Read the model definition and answer for the solid it produces. Units are mm, in the model's axes. A direction names the side the tool comes from. Coordinates: 2 decimals unless noted, no trailing zeros. Write each loop counter-clockwise with the first axis right and the second up, starting at its lowest first coordinate (ties: lowest second). Pieces come first, ordered by that corner, then holes. Notation, with made-up numbers: (-1.75, 30.5) -> (2.25, 30.5) arc R18 ccw to (2.25, 53.5) -> close; hole circle Ø4 at (-22, 39.5). An arc over 180 degrees is marked (long way). Answer as a JSON object with one key per item and string values. Group by question number.
(1) Find section D-D (x = 6.25). Give the vertices of the cut face in (y, z), then the cut area to 3 significant figures.
(2) Find section C-C (y = 3). Give the vertices of the cut face in (x, z), then the cut area to 3 significant figures.
(3) Find section B-B (x = -10). Give the vertices of the cut face in (y, z), then the cut area to 3 significant figures.
(4) Find section A-A (z = 18). Give the vertices of the cut face in (x, y).
(5) Flat-ended cylindrical pins translate along their axes: P1, Ø2, axis at x = 2.5, z = 11.5, coming from the +Y side; P2, Ø5, axis at x = 10, y = 3, coming from the +Z side. Find the tip coordinate at first contact, or state that the pin passes through.
(6) Straight lines are drawn through the part: L1, parallel to X at y = -12.65, z = 18; L2, parallel to Y at x = 10, z = 1.45; L3, parallel to Y at x = -5, z = 19.75. For each, find the intervals that lie inside material, in ascending order.
(7) Which of the six approach directions +Z, -Z, +X, -X, +Y, -Y give full straight-line access (tool end or side, diameter ignored) to faces 1 (the face through (0, 2, 3)), 2 (the face through (0, -13, 30))?
(8) For a pull along Z with two mould halves and no side action, classify faces 3 (the face through (0.21, -14.715, 0.301)), 4 (the face through (10.07, -13.48, 16.5)), 5 (the face through (0, -12, 17)), 6 (the face through (-9.93, -13.48, 16.5)) as +Z half, -Z half, draft (parallel to the pull), parting line (faces both ways), or undercut.
from build123d import *

# Parameters (mm, degrees)
SKETCH_1_W          = 30
SKETCH_1_H          = 30
EXTRUDE_1_DEPTH     = 3
SKETCH_2_R          = 1.5
CUT_EXTRUDE_1_DEPTH = 3.5
SKETCH_3_W          = 30
SKETCH_3_H          = 3
EXTRUDE_2_DEPTH     = 27
SKETCH_4_R          = 1.5
CUT_EXTRUDE_2_DEPTH = 27
FILLET_1_R          = 1
FILLET_2_R          = 1


with BuildPart() as part:
    # 草图1 → 凸台-拉伸1 (new body)
    with BuildSketch(Plane.XY):
        Rectangle(SKETCH_1_W, SKETCH_1_H)
    extrude(amount=EXTRUDE_1_DEPTH)

    # 草图2 → 切除-拉伸1 (cut)
    with BuildSketch(Plane.XY.offset(3)):
        with Locations((10, 3)):
            Circle(SKETCH_2_R)
        with Locations((-10, 3)):
            Circle(SKETCH_2_R)
    extrude(amount=-CUT_EXTRUDE_1_DEPTH, mode=Mode.SUBTRACT)

    # 草图3 → 凸台-拉伸2 (add)
    with BuildSketch(Plane.XY.offset(3)):
        with Locations((0, -13.5)):
            Rectangle(SKETCH_3_W, SKETCH_3_H)
    extrude(amount=EXTRUDE_2_DEPTH)

    # 草图4 → 切除-拉伸2 (cut)
    with BuildSketch(Plane(origin=(0, -12, 0), x_dir=(1, 0, 0), z_dir=(0, 1, 0))):
        with Locations(Location((10, -18, 0), (0, 0, 270))):
            Circle(SKETCH_4_R)
        with Locations(Location((-10, -18, 0), (0, 0, 270))):
            Circle(SKETCH_4_R)
    extrude(amount=-CUT_EXTRUDE_2_DEPTH, mode=Mode.SUBTRACT)

    # 圆角1
    fillet_1_edges = [part.edges().sort_by_distance(p)[0] for p in [
        (0, -12, 3),
    ]]
    fillet(fillet_1_edges, radius=FILLET_1_R)

    # 圆角2
    fillet_2_edges = [part.edges().sort_by_distance(p)[0] for p in [
        (0, -15, 0),
    ]]
    fillet(fillet_2_edges, radius=FILLET_2_R)


solid = part.part
Results below:
{
 "1": {"outline": "(-15, 1) arc R1 ccw to (-14, 0) -> (15, 0) -> (15, 3) -> (-11, 3) arc R1 cw to (-12, 4) -> (-12, 30) -> (-15, 30) -> close", "area": "171 mm2"},
 "2": {"outline": "(-15, 0) -> (-11.5, 0) -> (-11.5, 3) -> (-15, 3) -> close; (-8.5, 0) -> (8.5, 0) -> (8.5, 3) -> (-8.5, 3) -> close; (11.5, 0) -> (15, 0) -> (15, 3) -> (11.5, 3) -> close", "area": "72.0 mm2"},
 "3": {"outline": "(-15, 1) arc R1 ccw to (-14, 0) -> (1.5, 0) -> (1.5, 3) -> (-11, 3) arc R1 cw to (-12, 4) -> (-12, 16.5) -> (-15, 16.5) -> close; (-15, 19.5) -> (-12, 19.5) -> (-12, 30) -> (-15, 30) -> close; (4.5, 0) -> (15, 0) -> (15, 3) -> (4.5, 3) -> close", "area": "153 mm2"},
 "4": {"outline": "(-15, -15) -> (-11.5, -15) -> (-11.5, -12) -> (-15, -12) -> close; (-8.5, -15) -> (8.5, -15) -> (8.5, -12) -> (-8.5, -12) -> close; (11.5, -15) -> (15, -15) -> (15, -12) -> (11.5, -12) -> close"},
 "5": {"P1": "stops at y = -12", "P2": "stops at z = 3"},
 "6": {"L1": "x = -15 to -11.5, -8.5 to 8.5, 11.5 to 15", "L2": "y = -15 to 1.5, 4.5 to 15", "L3": "y = -15 to -12"},
 "7": {"face 1": "+Z, +X, -X, +Y", "face 2": "+Z, +X, -X, +Y, -Y"},
 "8": {"face 3": "-Z half", "face 4": "undercut", "face 5": "draft", "face 6": "undercut"}
}
